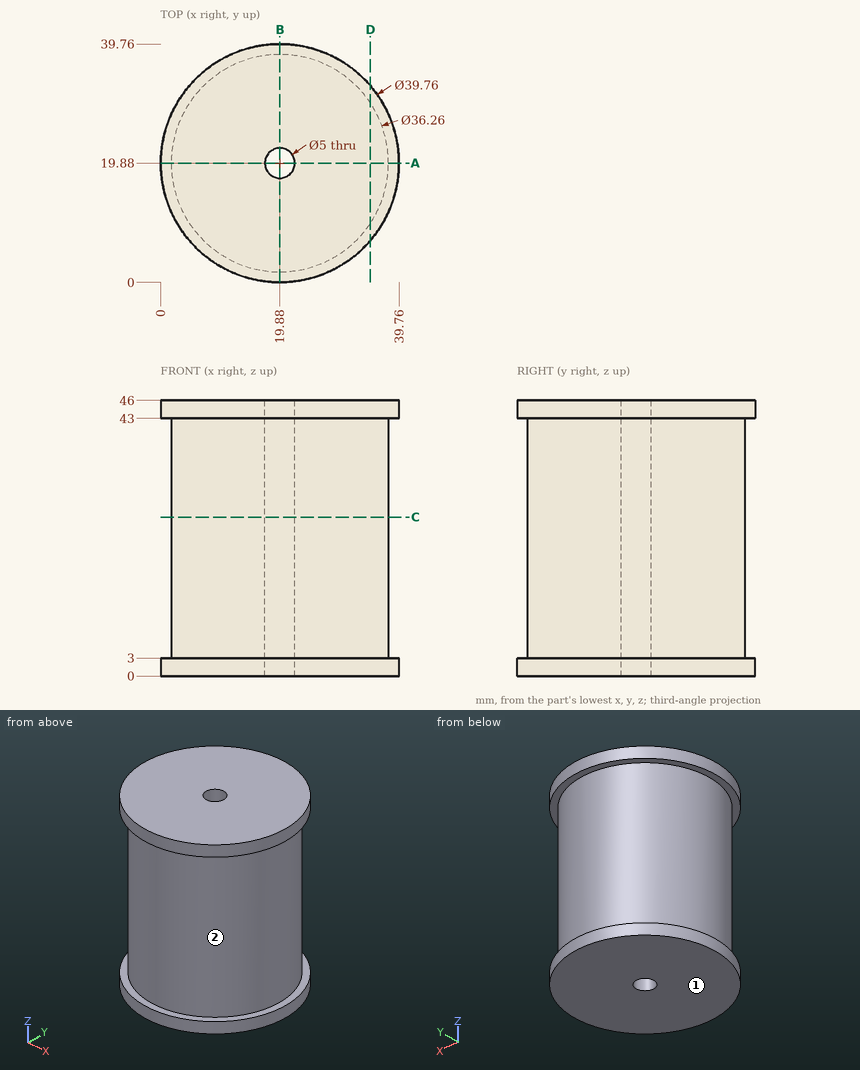
Job drawing, mm, ordinate dimensions from the low corner. One solid piece. A direction names the side the tool comes from. Give positions to 0.01 mm unless a question says otherwise; leave off trailing zeros. Write each loop counter-clockwise with the first axis right and the second up, starting at its lowest first coordinate (ties: lowest second). Pieces come first, ordered by that corner, then holes. Notation, with made-up numbers: (67.5, 13) - (98.5, 13) arc R10 cw to (98.5, 23) - close; hole circle Ø6 at (21.5, 9.25). An arc over 180 degrees is marked (long way). Use one line per item in the form item = value. Start each with the question number.
1. Band-saw the part on C-C on z = 26.5. Write the cut outline in (x, y).
2. Probe line 1 (Y direction, x = 19.88, z = 37); line 2 (X direction, y = 19, z = 36). List the from-to ranges inside material, lowest first. Write a range as [from, to].
3. Band-saw the part on D-D on x = 35. Write the cut outline in (y, z).
4. Band-saw the part on A-A on y = 19.88. Write the cut outline in (x, z).
5. 3-axis set-ups, long thin cutter, end or side, ignore diameter. For the marked faces 1 and 2: which of +Z, -Z, +X, -X, +Y, -Y reach the whole face in a straight line?
6. Drop flat-ended pins along their axis: pin 1 Ø12 at (x, z) = (5.5, 30) entering from +Y; pin 2 Ø3 at (x, y) = (6.5, 18) entering from -Z; pin 3 Ø1 at (y, z) = (15.5, 6.5) entering from +X; pin 4 Ø8 at (y, z) = (16, 5.5) entering from -X. Give the stop position or say it passes through.
Conclusion:
q1.outline = circle Ø36.26 at (19.88, 19.88); hole circle Ø5 at (19.88, 19.88)
q2.line_1 = [1.75, 17.38], [22.38, 38.01]
q2.line_2 = [1.77, 17.54], [22.22, 37.99]
q3.outline = (6.97, 0) - (32.79, 0) - (32.79, 3) - (29.88, 3) - (29.88, 43) - (32.79, 43) - (32.79, 46) - (6.97, 46) - (6.97, 43) - (9.88, 43) - (9.88, 3) - (6.97, 3) - close
q4.outline = (0, 0) - (17.38, 0) - (17.38, 46) - (0, 46) - (0, 43) - (1.75, 43) - (1.75, 3) - (0, 3) - close; (22.38, 0) - (39.76, 0) - (39.76, 3) - (38.01, 3) - (38.01, 43) - (39.76, 43) - (39.76, 46) - (22.38, 46) - close
q5.face_1 = -Z, +X, -X, +Y, -Y
q5.face_2 = none
q6.pin_1 = 35.96
q6.pin_2 = 0
q6.pin_3 = 37.59
q6.pin_4 = 0.01
